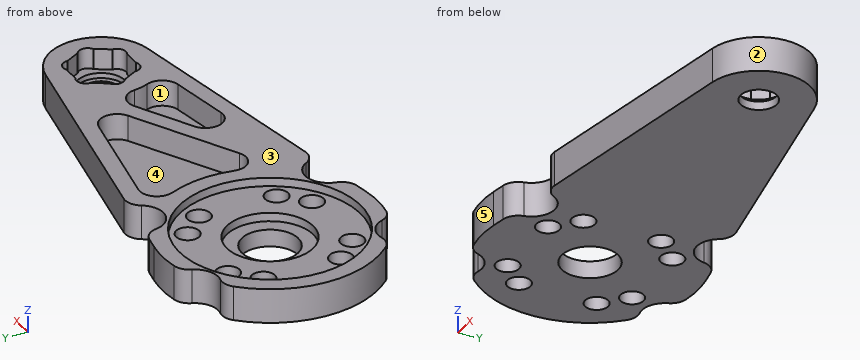
Autodesk Inventor part; units mm, degrees
ref_plane "YZ Plane" through (0, 0, 0) normal (1, 0, 0) x (0, 1, 0)
ref_plane "XZ Plane" through (0, 0, 0) normal (0, 1, 0) x (-1, 0, 0)
ref_plane "XY Plane" through (0, 0, 0) normal (0, 0, 1) x (1, 0, 0)
sketch "スケッチ1" plane through (0, 0, 0) normal (0, 0, 1) x (1, 0, 0)
  circle A0 centre (0, 0) radius 10.5 construction
  circle A1 centre (0, 0) radius 5 construction
  circle A2 centre (0, 0) radius 5.01
  circle A3 centre (0, 0) radius 10.51
  arc A4 (2.1531, 12.3132) -> (2.1531, -12.3132) centre (0, 0) ccw
  circle A5 centre (37.7359, 0) radius 2.75
  arc A6 (38.7694, -5.9103) -> (38.7694, 5.9103) centre (37.7359, 0) ccw
  line L0 (2.1531, 12.3132) -> (38.7694, 5.9103)
  line L1 (2.1531, -12.3132) -> (38.7694, -5.9103)
  line L2 (13.3804, 8.3196) -> (26.7879, 5.9751)
  line L3 (30.7947, -5.2745) -> (23.5904, -6.5342)
  arc A7 (2.1531, -12.3132) -> (-4.7001, 11.5827) centre (0, 0) ccw construction
  arc A8 (38.7694, 5.9103) -> (32.2717, -2.4783) centre (37.7359, 0) ccw construction
  line L4 (34.0196, 4.7105) -> (8.4896, -9.1748) construction
  line L5 (27.399, 2.248) -> (15.2168, -4.3777)
  line L6 (28.8431, 0.7568) -> (22.2903, -2.8072)
  line L7 (32.4358, 4.9875) -> (34.0196, 4.7105) construction
  line L8 (11.5743, -8.6354) -> (8.4896, -9.1748) construction
  arc A9 (31.783, -0.7501) -> (32.2717, -2.4783) centre (37.7359, 0) ccw
  arc A10 (12.2941, -2.2592) -> (11.2378, 5.4737) centre (0, 0) ccw
  line L9 (41.7889, 0) -> (41.2639, -0.9093) construction
  line L10 (39.7624, -3.51) -> (38.7124, -3.51) construction
  line L11 (35.7094, -3.51) -> (35.1844, -2.6007) construction
  line L12 (33.6829, 0) -> (34.2079, 0.9093) construction
  line L13 (35.7094, 3.51) -> (36.7594, 3.51) construction
  line L14 (39.7624, 3.51) -> (40.2874, 2.6007)
  arc A11 (41.2639, -0.9093) -> (41.2639, 0.9093) centre (40.7389, 0) ccw
  arc A12 (40.2874, 2.6007) -> (38.7124, 3.51) centre (39.2374, 2.6007) ccw
  arc A13 (36.7594, 3.51) -> (35.1844, 2.6007) centre (36.2344, 2.6007) ccw
  arc A14 (34.2079, 0.9093) -> (34.2079, -0.9093) centre (34.7329, 0) ccw
  arc A15 (35.1844, -2.6007) -> (36.7594, -3.51) centre (36.2344, -2.6007) ccw
  arc A16 (38.7124, -3.51) -> (40.2874, -2.6007) centre (39.2374, -2.6007) ccw
  line L15 (41.2639, -0.9093) -> (40.2874, -2.6007)
  line L16 (40.2874, -2.6007) -> (39.7624, -3.51) construction
  line L17 (38.7124, -3.51) -> (36.7594, -3.51)
  line L18 (36.7594, -3.51) -> (35.7094, -3.51) construction
  line L19 (35.1844, -2.6007) -> (34.2079, -0.9093)
  line L20 (34.2079, -0.9093) -> (33.6829, 0) construction
  line L21 (35.1844, 2.6007) -> (35.7094, 3.51) construction
  line L22 (34.2079, 0.9093) -> (35.1844, 2.6007)
  line L23 (36.7594, 3.51) -> (38.7124, 3.51)
  line L24 (38.7124, 3.51) -> (39.7624, 3.51) construction
  line L25 (40.2874, 2.6007) -> (41.2639, 0.9093)
  line L26 (41.2639, 0.9093) -> (41.7889, 0) construction
  circle A17 centre (37.7359, 0) radius 2.1
  circle A18 centre (0, 0) radius 3.275
  line L27 (0, 0) -> (27.1359, -16.96) construction
  line L28 (37.7359, 0) -> (27.1359, -16.96) construction
  line L29 (0, 0) -> (37.7359, 0) construction
  line L30 (0, 0) -> (0.848, -0.53)
  line L31 (8.003, 10.918) -> (-6.307, -11.978) construction
  arc A19 (-3.608, -11.968) -> (-7.826, -9.747) centre (-6.307, -11.978) ccw
  arc A20 (5.4321, 11.7398) -> (10.7002, 10.8186) centre (8.003, 10.918) ccw
  arc A21 (13.3804, 8.3196) -> (11.2378, 5.4737) centre (13.0359, 6.3495) ccw
  arc A22 (12.2941, -2.2592) -> (15.2168, -4.3777) centre (14.2612, -2.6207) ccw
  arc A23 (22.2903, -2.8072) -> (23.5904, -6.5342) centre (23.2459, -4.5641) ccw
  arc A24 (30.7947, -5.2745) -> (32.2717, -2.4783) centre (30.4502, -3.3043) ccw
  arc A25 (31.783, -0.7501) -> (28.8431, 0.7568) centre (29.7987, -1.0002) ccw
  arc A26 (27.399, 2.248) -> (26.7879, 5.9751) centre (26.4434, 4.005) ccw
  line L32 (8.003, -10.918) -> (-6.307, 11.978) construction
  arc A27 (-7.826, 9.747) -> (-3.608, 11.968) centre (-6.307, 11.978) ccw
  arc A28 (10.7002, -10.8186) -> (5.4321, -11.7398) centre (8.003, -10.918) ccw
  line L33 (-6.625, -10.6) -> (6.625, 10.6) construction
  circle A29 centre (4.505, 7.208) radius 1.35
  circle A30 centre (-7.208, 4.505) radius 1.35
  circle A31 centre (-4.505, -7.208) radius 1.35
  circle A32 centre (7.208, -4.505) radius 1.35
  circle A33 centre (4.505, -7.208) radius 1.35
  circle A34 centre (-7.208, -4.505) radius 1.35
  circle A35 centre (-4.505, 7.208) radius 1.35
  circle A36 centre (7.208, 4.505) radius 1.35
  circle A37 centre (-4.505, -7.208) radius 2.4 construction
  point P0 (8.4896, 9.1748)
  point P1 (34.0196, -4.7105)
  point P2 (10.3333, -7.0337)
  point P3 (32.3635, 2.6714)
  point P4 (39.7624, 3.51)
  point P5 (9.5861, 8.9831)
  point P6 (9.0332, 8.6401)
  point P7 (-3.608, 11.968)
  dimension "d0" = 21
  dimension "d1" = 10
  dimension "d2" = 0.01
  dimension "d3" = 0.01
  dimension "d4" = 25
  dimension "d7" = 5.5
  dimension "d8" = 6
  dimension "d15" = 2
  dimension "d16" = 2
  dimension "d17" = 1
  dimension "d18" = 1
  dimension "d20" = 1.05
  dimension "d23" = 360
  dimension "d25" = 7.02
  dimension "d30" = 4.2
  dimension "d33" = 6.55
  dimension "d41" = 20
  dimension "d42" = 32
  dimension "d46" = 27
  dimension "d47" = 1
  dimension "d48" = 90
  dimension "d49" = 2.699
  dimension "d50" = 2.699
  dimension "d51" = 2
  dimension "d52" = 2
  dimension "d53" = 2
  dimension "d55" = 2.699
  dimension "d56" = 2.699
  dimension "d57" = 2.7
  dimension "d58" = 8.5
  dimension "d61" = 360
  dimension "d63" = 4.8
extrude "押し出し1" add sketch "スケッチ1" along normal blind 4 contours L0 A20 A6 L1 A28 A4 A19 A27
extrude "押し出し2" add sketch "スケッチ1" along normal blind 1.6 contours A12 L14 | L14 L25 A11 L15 A16 L17 A15 L19 A14 L22 A13 L23 A12
extrude "押し出し3" add sketch "スケッチ1" along normal blind 1 contours A5
extrude "押し出し4" add sketch "スケッチ1" along normal blind 3 contours A3
extrude "押し出し5" add sketch "スケッチ1" along normal blind 2 contours A2
extrude "押し出し6" add sketch "スケッチ1" along normal blind 1 contours L2 A26 L5 A22 A10 A21 | L3 A23 L6 A25 A9 A24
fillet "フィレット1" radius 2 8 edges at (-3.608, -11.968, 2) (-7.826, -9.747, 2) (10.7002, 10.8186, 2) (5.4321, 11.7398, 2) (5.4321, -11.7398, 2) (10.7002, -10.8186, 2) (-7.826, 9.747, 2) (-3.608, 11.968, 2)
equation "\"d3\" = d2"
equation "\"d18\" = d17"
equation "\"d50\" = d49"
properties part number "Ankle_side_pitch_frame" material "アルミニウム 2014-T4"
The listing builds one solid part. Answer for the finished solid, in the listing's coordinates (mm). Face numbers are marked on the shaded views. A direction names the side the tool comes from. Give positions to 0.01 mm unless a question says otherwise; leave off trailing zeros. Write each loop counter-clockwise with the first axis right and the second up, starting at its lowest first coordinate (ties: lowest second). Pieces come first, ordered by that corner, then holes. Notation, with made-up numbers: (22.25, 88) - (61.25, 88) arc R19 cw to (61.25, 93) - close; hole circle Ø2 at (-3, 28.25). An arc over 180 degrees is marked (long way). One line per question, with ' | ' between items. Start each with the question number.
1. Section C-C, the plane y = 0 is taken. Count the separate pieces of the cut face and the enclosed holes in it, then the cut area to 3 significant figures.
2. Determine the mould class of the marked faces 3, 4 and 5 for opening direction Y: +Y half, -Y half, draft (parallel to the pull), parting line (faces both ways), or undercut.
3. Section A-A, the plane x = 0 is taken. Determine the outline of the cut face in (y, z) (3 decimals).
4. Section B-B, the plane x = 18 is taken. Determine the outline of the cut face in (y, z), then the cut area to 3 significant figures.
5. Given P1, Ø1.5, axis at y = -2, z = 2, coming from the -X side; P2, Ø1.5, axis at x = 30, z = 1, coming from the +Y side; P3, Ø1.5, axis at x = 2, z = 2.5, coming from the -Y side, each flat-ended and moving along its own axis, determine where each tip first touches the part or whether it passes through.
6. For the marked faces 1 and 2, determine the directions among +Z, -Z, +X, -X, +Y, -Y from which every point of the face is accessible in a straight line to the end or side of a thin tool.
7. Straight lines are drawn through the part: line 1 (Y direction, x = 0, z = 0.65) (3 decimals); line 2 (Y direction, x = 0, z = 2.4); line 3 (X direction, y = -1.25, z = 3.1). For each, find the intervals that lie inside material, in ascending order.
Result:
1) separate pieces: 3 | enclosed holes: 0 | area: 109 mm2
2) face 3: draft | face 4: undercut | face 5: -Y half
3) outline: (-12.5, 0) - (-3.275, 0) - (-3.275, 2) - (-5.01, 2) - (-5.01, 3) - (-10.51, 3) - (-10.51, 4) - (-12.5, 4) - close; (3.275, 0) - (12.5, 0) - (12.5, 4) - (10.51, 4) - (10.51, 3) - (5.01, 3) - (5.01, 2) - (3.275, 2) - close
4) outline: (-9.54, 0) - (9.54, 0) - (9.54, 4) - (7.51, 4) - (7.51, 1) - (-2.86, 1) - (-2.86, 4) - (-9.54, 4) - close | area: 45.2 mm2
5) P1: stops at x = -12.44 | P2: stops at y = 7.57 | P3: stops at y = -12.44
6) face 1: +Z | face 2: +Z, -Z, +X
7) line 1: y = -12.5 to -3.275, 3.275 to 12.5 | line 2: y = -12.5 to -5.01, 5.01 to 12.5 | line 3: x = -12.44 to -10.44, 10.44 to 12.44, 20.97 to 25.15, 31.87 to 34.4, 41.07 to 43.6
